```python
from build123d import *

# Parameters (mm, degrees)
F0_R     = 11
F1_DEPTH = 7


# Not quite as in the source:
# - a feature names something its author has since deleted; it is built from what else it names


with BuildPart() as f1:
    # F0 (on Top) → F1 (new body)
    with BuildSketch(Plane.XY):
        with BuildLine():
            Line((-15.0111069989, -4), (-12.9903810568, -7.5))
            ThreePointArc((-12.9903810568, -7.5), (-7.5, -12.9903810568), (0, -15))
            Line((0, -15), (4.0414518843, -15))
            Line((4.0414518843, -15), (-1.8747010448, -25.2470774586))
            ThreePointArc((-1.8747010448, -25.2470774586), (-1.5939696041, -26.9024559592), (-1.5, -28.5788383249))
            ThreePointArc((-1.5, -28.5788383249), (-2.0111126057, -32.4611240014), (-3.5096189432, -36.0788383249))
            Line((-3.5096189432, -36.0788383249), (8.6602540378, -15))
            Line((8.6602540378, -15), (33, -15))
            ThreePointArc((33, -15), (27.5227744249, -13.9642400438), (22.8019609728, -11))
            Line((22.8019609728, -11), (10.9696551146, -11))
            Line((10.9696551146, -11), (12.9903810568, -7.5))
            ThreePointArc((12.9903810568, -7.5), (15, 0), (12.9903810568, 7.5))
            Line((12.9903810568, 7.5), (10.9696551146, 11))
            Line((10.9696551146, 11), (22.8019609728, 11))
            ThreePointArc((22.8019609728, 11), (27.5227744249, 13.9642400438), (33, 15))
            Line((33, 15), (8.6602540378, 15))
            Line((8.6602540378, 15), (-3.5096189432, 36.0788383249))
            ThreePointArc((-3.5096189432, 36.0788383249), (-2.0111126057, 32.4611240014), (-1.5, 28.5788383249))
            ThreePointArc((-1.5, 28.5788383249), (-1.5939696041, 26.9024559592), (-1.8747010448, 25.2470774586))
            Line((-1.8747010448, 25.2470774586), (4.0414518843, 15))
            Line((4.0414518843, 15), (0, 15))
            ThreePointArc((0, 15), (-7.5, 12.9903810568), (-12.9903810568, 7.5))
            Line((-12.9903810568, 7.5), (-15.0111069989, 4))
            Line((-15.0111069989, 4), (-20.927259928, 14.2470774586))
            ThreePointArc((-20.927259928, 14.2470774586), (-25.8547738349, 16.8533018127), (-29.4903810568, 21.0788383249))
            Line((-29.4903810568, 21.0788383249), (-17.3205080757, 0))
            Line((-17.3205080757, 0), (-29.4903810568, -21.0788383249))
            ThreePointArc((-29.4903810568, -21.0788383249), (-25.8547738349, -16.8533018127), (-20.927259928, -14.2470774586))
            Line((-20.927259928, -14.2470774586), (-15.0111069989, -4))
        make_face()
        Circle(F0_R, mode=Mode.SUBTRACT)
        with BuildLine():
            Line((-26.0262794416, -23.0788383249), (-20.927259928, -14.2470774586))
            ThreePointArc((-20.927259928, -14.2470774586), (-25.8547738349, -16.8533018127), (-29.4903810568, -21.0788383249))
            ThreePointArc((-29.4903810568, -21.0788383249), (-24, -41.5692193817), (-3.5096189432, -36.0788383249))
            ThreePointArc((-3.5096189432, -36.0788383249), (-2.0111126057, -32.4611240014), (-1.5, -28.5788383249))
            ThreePointArc((-1.5, -28.5788383249), (-1.5939696041, -26.9024559592), (-1.8747010448, -25.2470774586))
            Line((-1.8747010448, -25.2470774586), (-6.9737205584, -34.0788383249))
            ThreePointArc((-6.9737205584, -34.0788383249), (-22, -38.1051177665), (-26.0262794416, -23.0788383249))
        make_face()
        with BuildLine():
            ThreePointArc((-3.5096189432, 36.0788383249), (-24, 41.5692193817), (-29.4903810568, 21.0788383249))
            ThreePointArc((-29.4903810568, 21.0788383249), (-25.8547738349, 16.8533018127), (-20.927259928, 14.2470774586))
            Line((-20.927259928, 14.2470774586), (-26.0262794416, 23.0788383249))
            ThreePointArc((-26.0262794416, 23.0788383249), (-22, 38.1051177665), (-6.9737205584, 34.0788383249))
            Line((-6.9737205584, 34.0788383249), (-1.8747010448, 25.2470774586))
            ThreePointArc((-1.8747010448, 25.2470774586), (-1.5939696041, 26.9024559592), (-1.5, 28.5788383249))
            ThreePointArc((-1.5, 28.5788383249), (-2.0111126057, 32.4611240014), (-3.5096189432, 36.0788383249))
        make_face()
        with BuildLine():
            ThreePointArc((22.8019609728, -11), (27.5227744249, -13.9642400438), (33, -15))
            ThreePointArc((33, -15), (43.6066017178, -10.6066017178), (48, 0))
            ThreePointArc((48, 0), (43.6066017178, 10.6066017178), (33, 15))
            ThreePointArc((33, 15), (27.5227744249, 13.9642400438), (22.8019609728, 11))
            Line((22.8019609728, 11), (33, 11))
            ThreePointArc((33, 11), (40.7781745931, 7.7781745931), (44, 0))
            ThreePointArc((44, 0), (40.7781745931, -7.7781745931), (33, -11))
            Line((33, -11), (22.8019609728, -11))
        make_face()
        with BuildLine():
            ThreePointArc((22.8019609728, 11), (18, 0), (22.8019609728, -11))
            Line((22.8019609728, -11), (33, -11))
            ThreePointArc((33, -11), (22, 0), (33, 11))
            Line((33, 11), (22.8019609728, 11))
        make_face()
        with BuildLine():
            Line((-26.0262794416, 23.0788383249), (-20.927259928, 14.2470774586))
            ThreePointArc((-20.927259928, 14.2470774586), (-9, 15.5884572681), (-1.8747010448, 25.2470774586))
            Line((-1.8747010448, 25.2470774586), (-6.9737205584, 34.0788383249))
            ThreePointArc((-6.9737205584, 34.0788383249), (-5.8748159108, 31.425847821), (-5.5, 28.5788383249))
            ThreePointArc((-5.5, 28.5788383249), (-13.6529905039, 17.9536542357), (-26.0262794416, 23.0788383249))
        make_face()
        with BuildLine():
            ThreePointArc((-1.8747010448, -25.2470774586), (-9, -15.5884572681), (-20.927259928, -14.2470774586))
            Line((-20.927259928, -14.2470774586), (-26.0262794416, -23.0788383249))
            ThreePointArc((-26.0262794416, -23.0788383249), (-13.6529905039, -17.9536542357), (-5.5, -28.5788383249))
            ThreePointArc((-5.5, -28.5788383249), (-5.8748159108, -31.425847821), (-6.9737205584, -34.0788383249))
            Line((-6.9737205584, -34.0788383249), (-1.8747010448, -25.2470774586))
        make_face()
    extrude(amount=F1_DEPTH)


solid = f1.part
```
Input: part model. Units: mm. Frame: model coordinates. A direction names the side the tool comes from. Give positions to 0.01 mm unless a question says otherwise; leave off trailing zeros. Order: outer loops, then holes, each group sorted by start corner. A loop starts at its lowest first (then second) coordinate and runs counter-clockwise, first axis right, second up. Notation, with made-up numbers: (75.25, 73.25) - (115.25, 73.25) arc R28 ccw to (115.25, 94.25) - close; hole circle Ø1 at (53.25, 34.25). An arc over 180 degrees is marked (long way). One line per item, written item: value.
1. Cut plane D-D, the plane y = -32. Output: boundary loops of the cut face in (x, z).
Determined:
outline: (-31.1, 0) - (-26.95, 0) - (-26.95, 7) - (-31.1, 7) - close; (-6.05, 0) - (-1.15, 0) - (-1.15, 7) - (-6.05, 7) - close
2. Cut plane A-A, the plane y = 2. Output: boundary loops of the cut face in (x, z).
Determined:
outline: (-18.48, 0) - (-10.82, 0) - (-10.82, 7) - (-18.48, 7) - close; (10.82, 0) - (14.87, 0) - (14.87, 7) - (10.82, 7) - close; (18.13, 0) - (22.18, 0) - (22.18, 7) - (18.13, 7) - close; (43.82, 0) - (47.87, 0) - (47.87, 7) - (43.82, 7) - close
3. Pin query (flat end, axial travel): pin 1 Ø4 at (y, z) = (6, 4) entering from +X; pin 2 Ø4 at (x, z) = (-0.5, 5.5) entering from -Y; pin 3 Ø1.2 at (x, z) = (1.5, 5) entering from +Y. Return the tip coordinate at first contact, or that it passes through.
Determined:
pin 1: x = 47.46
pin 2: y = -34.33
pin 3: y = 28.44
4. Draft query along Y for faces 1 (the face through (48, 0, 3)), 2 (the face through (21, 15, 3)), 3 (the face through (17, -11, 3)), 4 (the face through (-10, -6, 7)). Return one class per face: released by +Y, released by -Y, zero draft, split by the parting line, or undercut.
Determined:
face 1: split by the parting line
face 2: released by +Y
face 3: undercut
face 4: zero draft
5. Cut plane C-C, the plane z = 3. Give the number of separate pieces and of enclosed holes in the cut face, and give its area (3 significant figures).
Determined:
separate pieces: 1
enclosed holes: 7
area: 1,730 mm2
6. Reachability of faces 5 (the face through (-7.595, -12.935, 3.451)), 6 (the face through (-23.32, -10.39, 3.45)), 7 (the face through (-10, -6, 0)), 8 (the face through (21, -15, 3)) from +Z, -Z, +X, -X, +Y, -Y: full face, straight path, thin tool, end or side. Return the list, or none.
Determined:
face 5: +Z, -Z
face 6: +Z, -Z, -X
face 7: -Z, +X, -X, +Y, -Y
face 8: +Z, -Z, +X, -Y
7. Line query: probe 1 along Y at (x, z) = (-5, 2.5); probe 2 along X at (y, z) = (25, 5.25); probe 3 along X at (y, z) = (3.5, 6.5). Output: solid intervals per line, ascending.
Determined:
probe 1: -38.21 to -18.95, -14.14 to -9.8, 9.8 to 14.14, 18.95 to 38.21
probe 2: -31.07 to -26.9, -6.1 to -1.93, -1.73 to 2.89
probe 3: -19.34 to -10.43, 10.43 to 14.59, 18.41 to 22.57, 43.43 to 47.59
8. Cut plane B-B, the plane y = 12. Output: boundary loops of the cut face in (x, z).
Determined:
outline: (-24.25, 0) - (-19.63, 0) - (-19.63, 7) - (-24.25, 7) - close; (-9, 0) - (42, 0) - (42, 7) - (-9, 7) - close
